```python
from build123d import *

# Parameters (mm, degrees)
BOSS_EXTRUDE1_OUTLINE_R   = 7.9375
BOSS_EXTRUDE1_OUTLINE_R_2 = 6.4643
BOSS_EXTRUDE1_DEPTH       = 283.742530581
BOSS_EXTRUDE1_START       = -285
BOSS_EXTRUDE1_2_OUTLINE_W = 19
BOSS_EXTRUDE1_2_OUTLINE_H = 18
BOSS_EXTRUDE1_2_DEPTH     = 1.798021877
CUT_EXTRUDE1_DEPTH        = 9.525
CUT_EXTRUDE1_DEPTH_BACK   = 9.525


with BuildPart() as part:
    # Boss-Extrude1: read off the stored shape, not the designer's step
    # Boss-Extrude1 outline → Boss-Extrude1 (new body)
    with BuildSketch(Plane(origin=(0, 0, 0), x_dir=(1, 0, 0), z_dir=(0, 1, 0))):
        Circle(BOSS_EXTRUDE1_OUTLINE_R)
        Circle(BOSS_EXTRUDE1_OUTLINE_R_2, mode=Mode.SUBTRACT)
    extrude(amount=BOSS_EXTRUDE1_DEPTH)

    # Boss-Extrude1 2 outline → Boss-Extrude1 2 (cut)
    with BuildSketch(Plane(origin=(0, 0, 0), x_dir=(0.9992080363952592, 0.039790702470935205, 0), z_dir=(0.039790702470935205, -0.9992080363952592, 0)).offset(BOSS_EXTRUDE1_START)):
        with Locations((11.5, 0)):
            Rectangle(BOSS_EXTRUDE1_2_OUTLINE_W, BOSS_EXTRUDE1_2_OUTLINE_H)
    extrude(amount=BOSS_EXTRUDE1_2_DEPTH, mode=Mode.SUBTRACT)

    # Sketch2 → Cut-Extrude1 (cut, two sides: drawn at the far end of the back side and taken through both)
    with BuildSketch(Plane(origin=(0, 0, 0), x_dir=(0, 0, -1), z_dir=(1, 0, 0)).offset(-CUT_EXTRUDE1_DEPTH_BACK)):
        with BuildLine():
            Line((3.175, 284.215449167), (3.175, 258.815449167))
            ThreePointArc((3.175, 258.815449167), (0, 255.640449167), (-3.175, 258.815449167))
            Line((-3.175, 258.815449167), (-3.175, 284.215449167))
            Line((-3.175, 284.215449167), (3.175, 284.215449167))
        make_face()
    extrude(amount=CUT_EXTRUDE1_DEPTH + CUT_EXTRUDE1_DEPTH_BACK, mode=Mode.SUBTRACT)


solid = part.part
```
For this review, take the finished solid that the model builds, in its own axes (mm). Give positions to 0.01 mm unless a question says otherwise; leave off trailing zeros. Order: outer loops, then holes, each group sorted by start corner. A loop starts at its lowest first (then second) coordinate and runs counter-clockwise, first axis right, second up.
1) Take a section at A-A (z = 0). Give the boundary of the cut face in (x, y).
2) Wall thickness on line 1 (Z direction, x = 0, y = 155); line 2 (X direction, y = 13.5, z = -0.5): over which ranges is each line inside the solid? List them lowest first.
3) Take a section at C-C (y = 120). Give the boundary of the cut face in (x, z) (1 decimal), then the cut area to 3 significant figures.
4) The part is to be moulded in two halves that separate along Z. For faces 1 (the face through (-6.46, 139.84, -0.28)), 2 (the face through (-7.93, 139.87, -0.35)), 3 (the face through (-0.034, 283.425, 6.626)), say which applies: released by +Z, released by -Z, zero draft, split by the parting line, or undercut.
5) Insertion check: pin 1 (1.3 mm diameter, centred on x = 6.5, y = 273.5, fed in from -Z); pin 2 (0.8 mm diameter, centred on x = 6.5, y = 270.5, fed in from +Z); pin 3 (5 mm diameter, centred on x = -5, y = 41, fed in from +Z); pin 4 (6 mm diameter, centred on x = -2.5, z = -1, fed in from -Y). Each pin has a flat end and moves straight along its axis. Give the tip position at first contact, or say it passes through.
6) Take a section at B-B (x = -3). Give the boundary of the cut face in (y, z).
Derived:
1. outline: (-7.94, 0) - (-6.46, 0) - (-6.46, 255.64) - (-7.94, 255.64) - close; (6.46, 0) - (7.94, 0) - (7.94, 255.64) - (6.46, 255.64) - close
2. line 1: z = -7.94 to -6.46, 6.46 to 7.94
2. line 2: x = -7.92 to -6.44, 6.44 to 7.92
3. outline: circle Ø15.9 at (0, 0); hole circle Ø12.9 at (0, 0)
3. area: 66.7 mm2
4. face 1: undercut
4. face 2: split by the parting line
4. face 3: zero draft
5. pin 1: stops at z = -5.36
5. pin 2: stops at z = 5.08
5. pin 3: stops at z = 7.53
5. pin 4: passes through
6. outline: (0, -7.35) - (283.31, -7.35) - (283.31, -5.73) - (0, -5.73) - close; (0, 5.73) - (283.31, 5.73) - (283.31, 7.35) - (0, 7.35) - close
